Source: CAD feature listing. Evaluate the final solid. Frame: model axes, mm. A direction names the side the tool comes from. Give positions to 0.01 mm unless a question says otherwise; leave off trailing zeros. Loops run counter-clockwise (first coordinate to the right, second up) from the corner with the lowest first, then second, coordinate; pieces in that order, holes last.
```python
from build123d import *

# Parameters (mm, degrees)
F1_DEPTH  = 6.35
F2_W      = 60.7720911503
F2_H      = 40.4594867892
F1_FACE_W = 60.7720911503
F1_FACE_H = 6.35
F3_DEPTH  = 3.175
F5_DEPTH  = 25.4
F8_D      = 6.7564
F10_D     = 3.3


with BuildPart() as f1:
    # F0 (on Top) → F1 (new body)
    with BuildSketch(Plane.XY):
        with BuildLine():
            Line((0, -30.3860455751), (0, 0))
            Line((0, 0), (0, 30.3860455751))
            Line((0, 30.3860455751), (-6.4455037937, 30.3860455751))
            Line((-6.4455037937, 30.3860455751), (-6.4455037937, 24.0195686368))
            Line((-6.4455037937, 24.0195686368), (-12.811980732, 24.0195686368))
            Line((-12.811980732, 24.0195686368), (-12.811980732, 0))
            Line((-12.811980732, 0), (-12.811980732, -24.0195686368))
            ThreePointArc((-12.811980732, -24.0195686368), (-10.947282809, -28.5213476522), (-6.4455037937, -30.3860455751))
            Line((-6.4455037937, -30.3860455751), (0, -30.3860455751))
        make_face()
        with BuildLine():
            Line((-6.4455037937, 24.0195686368), (-6.4455037937, 30.3860455751))
            ThreePointArc((-6.4455037937, 30.3860455751), (-10.947282809, 28.5213476522), (-12.811980732, 24.0195686368))
            Line((-12.811980732, 24.0195686368), (-6.4455037937, 24.0195686368))
        make_face()
    extrude(amount=F1_DEPTH)

    # F2 (on Right) + F1_face (on face) → F3 (join)
    with BuildSketch(Plane.YZ):
        with Locations((0, 26.5797433946)):
            Rectangle(F2_W, F2_H)
        Polygon((-30.3860455751, 63.0933195353), (-30.3860455751, 46.8094867892), (30.3860455751, 46.8094867892), align=None)
    with BuildSketch(Plane(origin=(0, 0, 3.175), x_dir=(0, 1, 0), z_dir=(1, 0, 0))):
        Rectangle(F1_FACE_W, F1_FACE_H)
    extrude(amount=F3_DEPTH)

    # F4 (on face) → F5 (join)
    with BuildSketch(Plane.YZ.offset(3.175)):
        Polygon((-30.3860455751, 63.0933195353), (-30.3860455751, 56.7433195353), (30.3860455751, 40.4594867892), (30.3860455751, 46.8094867892), align=None)
    extrude(amount=F5_DEPTH)

    # F6: F1 across face


with BuildPart() as f1_1:
    add(f1.part)
    add(f1.part.mirror(Plane(origin=(28.575, 0, 51.7764031622), x_dir=(0, 1, 0), z_dir=(1, 0, 0))))

    # F8 (through all)
    with Locations(Plane(origin=(0, 12.1503507906, 45.3457264801), x_dir=(1, 0, 0), z_dir=(0, -0.2588190451, -0.9659258263))):
        with Locations((28.575, 12.5789687571)):
            Hole(F8_D / 2)

    # F10 (through all)
    with Locations(Plane(origin=(0, 0, 0), x_dir=(1, 0, 0), z_dir=(0, 0, -1))):
        with Locations((-6.4455037937, 24.0195686368), (-6.4455037937, -24.0195686368), (63.5955037937, -24.0195686368), (63.5955037937, 24.0195686368)):
            Hole(F10_D / 2)


solid = f1_1.part
```
(1) Reachability of faces 1 (the flat face through (0, 0, 29)), 2 (the flat face through (34.575, -0.425, 48.715)), 3 (the flat face through (64, 0, 6.35)) from +Z, -Z, +X, -X, +Y, -Y: full face, straight path, thin tool, end or side. Return the list, or none.
A:
face 1: +Z, -X, +Y, -Y
face 2: -Z, -Y
face 3: +Z, +X, +Y, -Y
(2) Section D-D, the plane y = 14.5. Return the cut outline in (x, z) (3 decimals), then the cut area to 3 significant figures.
A:
outline: (-12.812, 0) - (3.175, 0) - (3.175, 44.716) - (53.975, 44.716) - (53.975, 0) - (69.962, 0) - (69.962, 6.35) - (57.15, 6.35) - (57.15, 51.066) - (0, 51.066) - (0, 6.35) - (-12.812, 6.35) - close
area: 810 mm2
(3) First-contact query: pin 1 (6 mm diameter, centred on x = 15, y = 5.5, fed in from -Z); pin 2 (4 mm diameter, centred on x = 63, y = -14, fed in from +Z); pin 3 (17 mm diameter, centred on y = 1, z = 20.5, fed in from -X). Flat tips, straight axial feed; report the tip coordinate or a pass-through.
A:
pin 1: stops at z = 46.32
pin 2: stops at z = 6.35
pin 3: stops at x = 0
(4) Section A-A, the plane z = 16.5. Return the cut outline in (x, y) (3 decimals).
A:
outline: (0, -30.386) - (3.175, -30.386) - (3.175, 30.386) - (0, 30.386) - close; (53.975, -30.386) - (57.15, -30.386) - (57.15, 30.386) - (53.975, 30.386) - close
(5) Ray query, line 1 along X through (y, z) = (-16, 41) (3 decimals); line 2 along X through (y, z) = (23, 43.5); line 3 along Z through (x, y) = (62, -14). Return the intervals inside material, ascending.
A:
line 1: x = 0 to 3.175, 53.975 to 57.15
line 2: x = 0 to 57.15
line 3: z = 0 to 6.35
(6) Section B-B, the plane y = -21. Return the cut outline in (x, z) (3 decimals).
A:
outline: (-12.812, 0) - (3.175, 0) - (3.175, 54.228) - (53.975, 54.228) - (53.975, 0) - (69.962, 0) - (69.962, 6.35) - (57.15, 6.35) - (57.15, 60.578) - (0, 60.578) - (0, 6.35) - (-12.812, 6.35) - close
(7) Mould query, pull axis Y, two halves, no side actions, for faces 4 (the cylindrical face through (-11, -28.47, 3.13)), 5 (the cylindrical face through (68.05, 28.57, 3.13)), 6 (the cylindrical face through (-5.229, 22.904, 3.219)). Classes: pulls with the +Y half, pulls with the -Y half, needs draft (parallel to the pull), parting line crosses it, or undercut.
A:
face 4: pulls with the -Y half
face 5: pulls with the +Y half
face 6: undercut
(8) Section C-C, the plane x = 37. Return the cut outline in (y, z), then the cut area to 3 significant figures.
A:
outline: (-30.39, 56.74) - (30.39, 40.46) - (30.39, 46.81) - (-30.39, 63.09) - close
area: 386 mm2
